Geometry: final body of the model. Coordinates: model frame, mm. Coordinates: 2 decimals unless noted, no trailing zeros. Order: outer loops, then holes, each group sorted by start corner. A loop starts at its lowest first (then second) coordinate and runs counter-clockwise, first axis right, second up. Notation, with made-up numbers: M 35.5,13.5 L 54.5,13.5 A26 cw 54.5,33.5 Z; hole C 76,35.5 d11. An arc over 180 degrees is marked long. One line per question, with ' | ' between items.
from build123d import *

# Parameters (mm, degrees)
SKETCH1_R           = 40
SKETCH1_R_2         = 2
SKETCH1_W           = 15.6
SKETCH1_H           = 5.6
SKETCH1_W_2         = 5.6
SKETCH1_H_2         = 20.6
SKETCH1_W_3         = 10.6
BOSS_EXTRUDE1_DEPTH = 5


with BuildPart() as part:
    # Sketch1 → Boss-Extrude1 (new body)
    with BuildSketch(Plane(origin=(0, 0, 0), x_dir=(-1, 0, 0), z_dir=(0, -1, 0))):
        with BuildLine():
            Line((-144.276672243, 28.966950724), (-144.276672243, -46.033049276))
            Line((-144.276672243, -46.033049276), (-185.693858461, -46.033049276))
            ThreePointArc((-185.693858461, -46.033049276), (-70.476672243, -223.033049276), (44.740513975, -46.033049276))
            Line((44.740513975, -46.033049276), (3.323327757, -46.033049276))
            Line((3.323327757, -46.033049276), (3.323327757, 28.966950724))
            Line((3.323327757, 28.966950724), (3.323327757, 33.966950724))
            Line((3.323327757, 33.966950724), (-15.476672243, 33.966950724))
            Line((-15.476672243, 33.966950724), (-15.476672243, 28.966950724))
            Line((-15.476672243, 28.966950724), (-30.476672243, 28.966950724))
            Line((-30.476672243, 28.966950724), (-30.476672243, 33.966950724))
            Line((-30.476672243, 33.966950724), (-110.476672243, 33.966950724))
            Line((-110.476672243, 33.966950724), (-110.476672243, 28.966950724))
            Line((-110.476672243, 28.966950724), (-125.476672243, 28.966950724))
            Line((-125.476672243, 28.966950724), (-125.476672243, 33.966950724))
            Line((-125.476672243, 33.966950724), (-144.276672243, 33.966950724))
            Line((-144.276672243, 33.966950724), (-144.276672243, 28.966950724))
        make_face()
        with Locations(Location((-70.476672243, -11.033049276, 0), (0, 0, 90))):
            Circle(SKETCH1_R, mode=Mode.SUBTRACT)
        with Locations(Location((-34.976672243, 24.466950724, 0), (0, 0, 90))):
            Circle(SKETCH1_R_2, mode=Mode.SUBTRACT)
        with Locations(Location((-105.976672243, 24.466950724, 0), (0, 0, 90))):
            Circle(SKETCH1_R_2, mode=Mode.SUBTRACT)
        with Locations(Location((-105.976672243, -46.533049276, 0), (0, 0, 90))):
            Circle(SKETCH1_R_2, mode=Mode.SUBTRACT)
        with Locations(Location((-34.976672243, -46.533049276, 0), (0, 0, 90))):
            Circle(SKETCH1_R_2, mode=Mode.SUBTRACT)
        Polygon((-20.176672243, -6.333049276), (-20.176672243, -1.333049276), (-15.176672243, -1.333049276), (-15.176672243, 14.266950724), (-20.176672243, 14.266950724), (-20.176672243, 19.266950724), (-25.776672243, 19.266950724), (-25.776672243, -6.333049276), align=None, mode=Mode.SUBTRACT)
        Polygon((-20.176672243, -25.733049276), (-20.176672243, -30.733049276), (-15.176672243, -30.733049276), (-15.176672243, -46.333049276), (-20.176672243, -46.333049276), (-20.176672243, -51.333049276), (-25.776672243, -51.333049276), (-25.776672243, -25.733049276), align=None, mode=Mode.SUBTRACT)
        Polygon((-120.776672243, -6.333049276), (-115.176672243, -6.333049276), (-115.176672243, 19.266950724), (-120.776672243, 19.266950724), (-120.776672243, 14.266950724), (-125.776672243, 14.266950724), (-125.776672243, -1.333049276), (-120.776672243, -1.333049276), align=None, mode=Mode.SUBTRACT)
        Polygon((-120.776672243, -25.733049276), (-115.176672243, -25.733049276), (-115.176672243, -51.333049276), (-120.776672243, -51.333049276), (-120.776672243, -46.333049276), (-125.776672243, -46.333049276), (-125.776672243, -30.733049276), (-120.776672243, -30.733049276), align=None, mode=Mode.SUBTRACT)
        with Locations((-7.976672243, -69.533049276)):
            Rectangle(SKETCH1_W, SKETCH1_H, mode=Mode.SUBTRACT)
        with Locations((17.023327757, -92.033049276)):
            Rectangle(SKETCH1_W_2, SKETCH1_H_2, mode=Mode.SUBTRACT)
        with Locations((17.023327757, -137.033049276)):
            Rectangle(SKETCH1_W_2, SKETCH1_H_2, mode=Mode.SUBTRACT)
        with Locations((-7.976672243, -159.533049276)):
            Rectangle(SKETCH1_W, SKETCH1_H, mode=Mode.SUBTRACT)
        with Locations((-32.976672243, -137.033049276)):
            Rectangle(SKETCH1_W_2, SKETCH1_H_2, mode=Mode.SUBTRACT)
        with Locations((-32.976672243, -92.033049276)):
            Rectangle(SKETCH1_W_2, SKETCH1_H_2, mode=Mode.SUBTRACT)
        with Locations((-37.976672243, -204.533049276)):
            Rectangle(SKETCH1_W, SKETCH1_H, mode=Mode.SUBTRACT)
        Polygon((-20.776672243, -176.733049276), (-20.776672243, -181.733049276), (-25.776672243, -181.733049276), (-25.776672243, -187.333049276), (-20.776672243, -187.333049276), (-20.776672243, -192.333049276), (-15.176672243, -192.333049276), (-15.176672243, -187.333049276), (-10.176672243, -187.333049276), (-10.176672243, -181.733049276), (-15.176672243, -181.733049276), (-15.176672243, -176.733049276), align=None, mode=Mode.SUBTRACT)
        with Locations((-102.976672243, -204.533049276)):
            Rectangle(SKETCH1_W, SKETCH1_H, mode=Mode.SUBTRACT)
        Polygon((-120.176672243, -176.733049276), (-125.776672243, -176.733049276), (-125.776672243, -181.733049276), (-130.776672243, -181.733049276), (-130.776672243, -187.333049276), (-125.776672243, -187.333049276), (-125.776672243, -192.333049276), (-120.176672243, -192.333049276), (-120.176672243, -187.333049276), (-115.176672243, -187.333049276), (-115.176672243, -181.733049276), (-120.176672243, -181.733049276), align=None, mode=Mode.SUBTRACT)
        with Locations((-125.476672243, -159.533049276)):
            Rectangle(SKETCH1_W_3, SKETCH1_H, mode=Mode.SUBTRACT)
        with Locations((-155.476672243, -159.533049276)):
            Rectangle(SKETCH1_W_3, SKETCH1_H, mode=Mode.SUBTRACT)
        with Locations((-107.976672243, -137.033049276)):
            Rectangle(SKETCH1_W_2, SKETCH1_H_2, mode=Mode.SUBTRACT)
        with Locations((-172.976672243, -137.033049276)):
            Rectangle(SKETCH1_W_2, SKETCH1_H_2, mode=Mode.SUBTRACT)
        with Locations((-172.976672243, -92.033049276)):
            Rectangle(SKETCH1_W_2, SKETCH1_H_2, mode=Mode.SUBTRACT)
        with Locations((-107.976672243, -92.033049276)):
            Rectangle(SKETCH1_W_2, SKETCH1_H_2, mode=Mode.SUBTRACT)
        with Locations((-125.476672243, -69.533049276)):
            Rectangle(SKETCH1_W_3, SKETCH1_H, mode=Mode.SUBTRACT)
        with Locations((-155.476672243, -69.533049276)):
            Rectangle(SKETCH1_W_3, SKETCH1_H, mode=Mode.SUBTRACT)
    extrude(amount=BOSS_EXTRUDE1_DEPTH)


solid = part.part
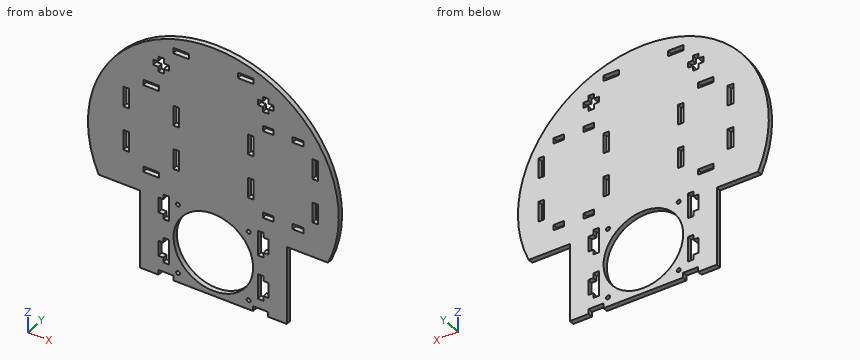
1. Section D-D, the plane y = -2.1. Give the number of separate pieces and of enclosed holes in the cut face, and give its area (3 significant figures).
Response values:
separate pieces: 1 | enclosed holes: 27 | area: 41,300 mm^2
2. Material intervals for line 1 (X direction, y = -1.45, z = 31); line 2 (X direction, y = -4.35, z = 38); line 3 (X direction, y = -2.75, z = 138.5), sorted ascending. Write a range as [from, to].
Response values:
line 1: x = [-3.32, 15.18], [25.78, 35.82], [105.14, 115.18], [125.78, 144.28] | line 2: x = [-3.32, 15.18], [25.78, 40.93], [100.02, 115.18], [125.78, 144.28] | line 3: x = [-48.5, -19.82], [-14.22, 30.18], [35.78, 105.18], [110.78, 170.18], [175.78, 189.46]
3. Section B-B, the plane z = 13.5. Output: boundary loops of the cut face in (x, y), and give its area (3 significant figures).
Response values:
outline: M -3.32,-5 L 30.55,-5 L 30.55,0 L -3.32,0 Z; M 110.4,-5 L 144.28,-5 L 144.28,0 L 110.4,0 Z | area: 339 mm^2
4. Pin query (flat end, axial travel): P1, Ø2.5, axis at x = 104.5, y = -2, coming from the +Z side; P2, Ø1.5, axis at y = -2, z = 69, coming from the -X side; P3, Ø2, axis at y = -1.5, z = 24.5, coming from the +X side. Return the tip coordinate at first contact, or that it passes through.
Response values:
P1: stops at z = 218.7 | P2: stops at x = -52.53 | P3: stops at x = 144.28
5. Section C-C, the plane x = 81.5. Output: boundary loops of the cut face in (y, z).
Response values:
outline: M -5,-33.97 L 0,-33.97 L 0,-27.42 L -5,-27.42 Z; M -5,49.48 L 0,49.48 L 0,222.55 L -5,222.55 Z
6. Section A-A, the plane x = 153.5. Output: boundary loops of the cut face in (y, z), and give its area (3 significant figures).
Response values:
outline: M -5,46.03 L 0,46.03 L 0,66.73 L -5,66.73 Z; M -5,72.33 L 0,72.33 L 0,156.73 L -5,156.73 Z; M -5,162.33 L 0,162.33 L 0,191.81 L -5,191.81 Z | area: 673 mm^2
